The listing builds one solid part. Answer for the finished solid, in the listing's coordinates (mm). Face numbers are marked on the shaded views. A direction names the side the tool comes from. Round coordinates to 2 decimals unless told otherwise and drop trailing zeros. Loops run counter-clockwise (first coordinate to the right, second up) from the corner with the lowest first, then second, coordinate; pieces in that order, holes last. Notation, with made-up numbers: (-26.75, -26) -> (-3.75, -26) arc R15 cw to (-3.75, -1) -> close; hole circle Ø2 at (83, 52.5). An arc over 180 degrees is marked (long way). Use a Markdown table: item, result. Add a question column.
Q1. Section D-D on y = 15.5 is taken. Give the vertices of the cut face in (x, z), then the cut area to 3 significant figures.
Q2. Section C-C on x = 49 is taken. Give the vertices of the cut face in (y, z), then the cut area to 3 significant figures.
Q3. Section B-B on y = 21 is taken. Give the vertices of the cut face in (x, z).
Q4. Which of the six approach directions +Z, -Z, +X, -X, +Y, -Y give full straight-line access (tool end or side, diameter ignored) to the marked faces 1 and 2?
Q5. Section A-A on z = -21 is taken. Give the vertices of the cut face in (x, y).
Q6. Given pin 1 Ø3.5 at (y, z) = (5.5, -5.5) entering from +X; pin 2 Ø8 at (x, y) = (60, 23) entering from +Z; pin 3 Ø0.6 at (y, z) = (23.5, -21.5) entering from +X; pin 4 Ø10 at (x, z) = (54, -5) entering from +Y, each flat-ended and moving along its own axis, determine where each tip first touches the part or whether it passes through.
Q7. Consider line 1 (Y direction, x = 44.85, z = -5.5); line 2 (Z direction, x = 45.7, y = 5.5); line 3 (Z direction, x = 44, y = 36). Determine where each line is inside the solid, lowest interval first.
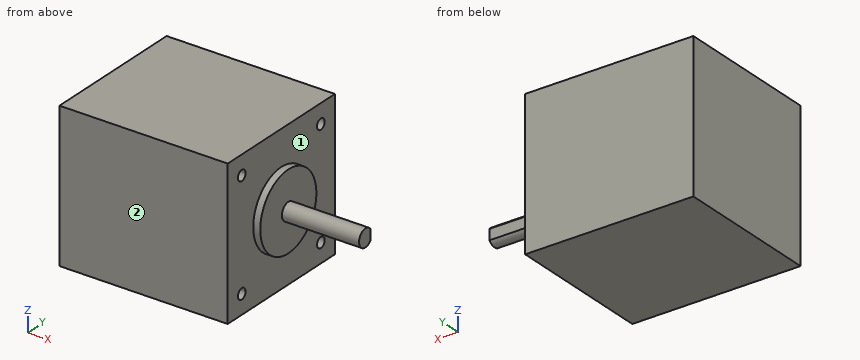
from build123d import *

# Parameters (mm, degrees)
SKETCH1_W           = 42
SKETCH1_H           = 42
BOSS_EXTRUDE1_DEPTH = 48
SKETCH3_R           = 11
BOSS_EXTRUDE2_DEPTH = 2
SKETCH4_R           = 2.5
BOSS_EXTRUDE3_DEPTH = 22
SKETCH5_W           = 15
SKETCH5_H           = 9.626973265
CUT_EXTRUDE1_DEPTH  = 2
CUT_EXTRUDE2_DEPTH  = 4.5


with BuildPart() as part:
    # Sketch1 → Boss-Extrude1 (new body)
    with BuildSketch(Plane(origin=(0, 0, 0), x_dir=(0, 0, -1), z_dir=(1, 0, 0))):
        with Locations((21, 21)):
            Rectangle(SKETCH1_W, SKETCH1_H)
    extrude(amount=BOSS_EXTRUDE1_DEPTH)

    # Sketch3 → Boss-Extrude2 (add)
    with BuildSketch(Plane(origin=(48, 0, 0), x_dir=(0, 0, -1), z_dir=(1, 0, 0))):
        with Locations(Location((21, 21, 0), (0, 0, 180))):
            Circle(SKETCH3_R)
    extrude(amount=BOSS_EXTRUDE2_DEPTH)

    # Sketch4 → Boss-Extrude3 (add)
    with BuildSketch(Plane(origin=(50, 0, 0), x_dir=(0, 0, -1), z_dir=(1, 0, 0))):
        with Locations((21, 21)):
            Circle(SKETCH4_R)
    extrude(amount=BOSS_EXTRUDE3_DEPTH)

    # Sketch5 → Cut-Extrude1 (cut)
    with BuildSketch(Plane(origin=(0, 23, 0), x_dir=(1, 0, 0), z_dir=(0, 1, 0))):
        with Locations((64.5, 20.688698753)):
            Rectangle(SKETCH5_W, SKETCH5_H)
    extrude(amount=CUT_EXTRUDE1_DEPTH, mode=Mode.SUBTRACT)

    # Sketch6 → Cut-Extrude2 (cut)
    with BuildSketch(Plane(origin=(48, 0, 0), x_dir=(0, 0, -1), z_dir=(1, 0, 0))):
        with BuildLine():
            Line((5.5, 35), (5.5, 36.5))
            Line((5.5, 36.5), (7, 36.5))
            ThreePointArc((7, 36.5), (4.439339828, 37.560660172), (5.5, 35))
        make_face()
        with BuildLine():
            Line((7, 36.5), (5.5, 36.5))
            Line((5.5, 36.5), (5.5, 35))
            ThreePointArc((5.5, 35), (6.560660172, 35.439339828), (7, 36.5))
        make_face()
        with BuildLine():
            ThreePointArc((38, 36.5), (36.5, 38), (35, 36.5))
            Line((35, 36.5), (36.5, 36.5))
            Line((36.5, 36.5), (36.5, 35))
            ThreePointArc((36.5, 35), (37.560660172, 35.439339828), (38, 36.5))
        make_face()
        with BuildLine():
            Line((36.5, 36.5), (35, 36.5))
            ThreePointArc((35, 36.5), (35.439339828, 35.439339828), (36.5, 35))
            Line((36.5, 35), (36.5, 36.5))
        make_face()
        with BuildLine():
            ThreePointArc((38, 5.5), (37.560660172, 6.560660172), (36.5, 7))
            Line((36.5, 7), (36.5, 5.5))
            Line((36.5, 5.5), (35, 5.5))
            ThreePointArc((35, 5.5), (36.5, 4), (38, 5.5))
        make_face()
        with BuildLine():
            Line((36.5, 5.5), (36.5, 7))
            ThreePointArc((36.5, 7), (35.439339828, 6.560660172), (35, 5.5))
            Line((35, 5.5), (36.5, 5.5))
        make_face()
        with BuildLine():
            ThreePointArc((7, 5.5), (6.560660172, 6.560660172), (5.5, 7))
            Line((5.5, 7), (5.5, 5.5))
            Line((5.5, 5.5), (7, 5.5))
        make_face()
        with BuildLine():
            Line((5.5, 5.5), (5.5, 7))
            ThreePointArc((5.5, 7), (4.439339828, 4.439339828), (7, 5.5))
            Line((7, 5.5), (5.5, 5.5))
        make_face()
    extrude(amount=-CUT_EXTRUDE2_DEPTH, mode=Mode.SUBTRACT)


solid = part.part
Checked values:
| question | item | result |
|---|---|---|
| 1 | outline | (0, -42) -> (48, -42) -> (48, -30.53) -> (50, -30.53) -> (50, -11.47) -> (48, -11.47) -> (48, 0) -> (0, 0) -> close |
| 1 | area | 2,050 mm2 |
| 2 | outline | circle Ø22 at (21, -21) |
| 2 | area | 380 mm2 |
| 3 | outline | (0, -42) -> (48, -42) -> (48, -32) -> (50, -32) -> (50, -23.5) -> (72, -23.5) -> (72, -18.5) -> (50, -18.5) -> (50, -10) -> (48, -10) -> (48, 0) -> (0, 0) -> close |
| 4 | face 1 | +X |
| 4 | face 2 | +Z, -Z, +X, -X, -Y |
| 5 | outline | (0, 0) -> (48, 0) -> (48, 10) -> (50, 10) -> (50, 18.5) -> (72, 18.5) -> (72, 23) -> (57, 23) -> (57, 23.5) -> (50, 23.5) -> (50, 32) -> (48, 32) -> (48, 42) -> (0, 42) -> close |
| 6 | pin 1 | stops at x = 48 |
| 6 | pin 2 | stops at z = -18.5 |
| 6 | pin 3 | stops at x = 57 |
| 6 | pin 4 | passes through |
| 7 | line 1 | y = 0 to 4, 7 to 35, 38 to 42 |
| 7 | line 2 | z = -42 to -38, -35 to -7, -4 to 0 |
| 7 | line 3 | z = -42 to -37.91, -35.09 to -6.91, -4.09 to 0 |
